Source: CAD feature listing. Evaluate the final solid. Frame: model axes, mm. Coordinates: 2 decimals unless noted, no trailing zeros. Write each loop counter-clockwise with the first axis right and the second up, starting at its lowest first coordinate (ties: lowest second). Pieces come first, ordered by that corner, then holes. Notation, with made-up numbers: (83.25, 74.25) -> (129.25, 74.25) arc R20 cw to (129.25, 80.25) -> close; hole circle Ø7 at (-5, 88). An arc over 180 degrees is marked (long way). One line per item, written item: value. Start each with the question number.
1. Section query B-B, the plane y = 25. Output: boundary loops of the cut face in (x, z), and give its area (3 significant figures).
2. Section query A-A, the plane x = 30. Output: boundary loops of the cut face in (y, z).
3. Section query C-C, the plane x = 20.5. Output: boundary loops of the cut face in (y, z).
4. Line query: line 1 (Y direction, x = 30, z = 8.5); line 2 (Y direction, x = 40, z = 5.25); line 3 (Y direction, x = 62.5, z = 8.5). Output: solid intervals per line, ascending.
from build123d import *

# Parameters (mm, degrees)
SKETCH_W  = 65
SKETCH_H  = 40
SKETCH_R  = 1.5625
PAD_DEPTH = 12
FILLET_R  = 3


with BuildPart() as part:
    # Sketch → Pad (new body)
    with BuildSketch(Plane.XY):
        with Locations((32.5, 20)):
            Rectangle(SKETCH_W, SKETCH_H)
        with Locations((20, 25)):
            Circle(SKETCH_R, mode=Mode.SUBTRACT)
        with Locations((40, 25)):
            Circle(SKETCH_R, mode=Mode.SUBTRACT)
        with Locations((30, 15)):
            Circle(SKETCH_R, mode=Mode.SUBTRACT)
        with Locations((50, 15)):
            Circle(SKETCH_R, mode=Mode.SUBTRACT)
    extrude(amount=PAD_DEPTH)

    # Fillet
    fillet_edges = [part.edges().sort_by_distance(p)[0] for p in [
        (65, 40, 6),
        (0, 40, 6),
        (0, 0, 6),
        (65, 0, 6),
    ]]
    fillet(fillet_edges, radius=FILLET_R)


solid = part.part
Computed values:
1. outline: (0, 0) -> (18.44, 0) -> (18.44, 12) -> (0, 12) -> close; (21.56, 0) -> (38.44, 0) -> (38.44, 12) -> (21.56, 12) -> close; (41.56, 0) -> (65, 0) -> (65, 12) -> (41.56, 12) -> close
1. area: 705 mm²
2. outline: (0, 0) -> (13.44, 0) -> (13.44, 12) -> (0, 12) -> close; (16.56, 0) -> (40, 0) -> (40, 12) -> (16.56, 12) -> close
3. outline: (0, 0) -> (23.52, 0) -> (23.52, 12) -> (0, 12) -> close; (26.48, 0) -> (40, 0) -> (40, 12) -> (26.48, 12) -> close
4. line 1: y = 0 to 13.44, 16.56 to 40
4. line 2: y = 0 to 23.44, 26.56 to 40
4. line 3: y = 0.04 to 39.96
